Here's how the part is built. I have some questions about the finished solid (model axes, mm). A direction names the side the tool comes from. Give positions to 0.01 mm unless a question says otherwise; leave off trailing zeros. Loops run counter-clockwise (first coordinate to the right, second up) from the corner with the lowest first, then second, coordinate; pieces in that order, holes last. Notation, with made-up numbers: (57, 82.5) - (76, 82.5) arc R22 ccw to (76, 99.5) - close; hole circle Ø1 at (39, 74). An arc over 180 degrees is marked (long way). Use one line per item in the form item = value.
from build123d import *

# Parameters (mm, degrees)
SKETCH1_W           = 20
SKETCH1_H           = 60
BOSS_EXTRUDE1_DEPTH = 5
SKETCH2_W           = 20
SKETCH2_H           = 13
BOSS_EXTRUDE2_DEPTH = 4.5
SKETCH3_W           = 15
SKETCH3_H           = 6.5
CUT_EXTRUDE1_DEPTH  = 14
CUT_EXTRUDE2_DEPTH  = 10


with BuildPart() as part:
    # Sketch1 → Boss-Extrude1 (new body)
    with BuildSketch(Plane.XY):
        with Locations((10, 30)):
            Rectangle(SKETCH1_W, SKETCH1_H)
    extrude(amount=BOSS_EXTRUDE1_DEPTH)

    # Sketch2 → Boss-Extrude2 (add)
    with BuildSketch(Plane.XY.offset(5)):
        with Locations((10, 6.5)):
            Rectangle(SKETCH2_W, SKETCH2_H)
    extrude(amount=BOSS_EXTRUDE2_DEPTH)

    # Sketch3 → Cut-Extrude1 (cut, through all)
    with BuildSketch(Plane(origin=(0, 13, 0), x_dir=(1, 0, 0), z_dir=(0, 1, 0))):
        with Locations((10, -5.25)):
            Rectangle(SKETCH3_W, SKETCH3_H)
    extrude(amount=-CUT_EXTRUDE1_DEPTH, mode=Mode.SUBTRACT)

    # Sketch4 → Cut-Extrude2 (cut)
    with BuildSketch(Plane.XY.offset(5)):
        with BuildLine():
            Line((11.75, 54), (11.75, 18))
            ThreePointArc((11.75, 18), (10, 16.25), (8.25, 18))
            Line((8.25, 18), (8.25, 54))
            ThreePointArc((8.25, 54), (10, 55.75), (11.75, 54))
        make_face()
    extrude(amount=-CUT_EXTRUDE2_DEPTH, mode=Mode.SUBTRACT)


solid = part.part
(1) For faces 1 (the cylindrical face through (9.96, 55.75, 2.54)), 2 (the flat face through (10, 7, 8.5)), 3 (the flat face through (2.5, 7, 5)), which set-ups out of +Z, -Z, +X, -X, +Y, -Y let a thin tool reach every point of the face, with its end or its side?
Geometry says:
face_1 = +Z, -Z
face_2 = +Y, -Y
face_3 = -Y
(2) If I drill on probe 1 along X at (y, z) = (6.5, 3); probe 2 along X at (y, z) = (41, 0.5); probe 3 along Z at (x, y) = (8, 5), over which ranges is the centre line in solid material (lowest first)?
Geometry says:
probe_1 = 0 to 2.5, 17.5 to 20
probe_2 = 0 to 8.25, 11.75 to 20
probe_3 = 0 to 2, 8.5 to 9.5
(3) If we section it at C-C (y = 52): List the corners of the cut face in (x, z) for me, plus the area to 3 significant figures.
Geometry says:
outline = (0, 0) - (8.25, 0) - (8.25, 5) - (0, 5) - close; (11.75, 0) - (20, 0) - (20, 5) - (11.75, 5) - close
area = 82.5 mm²
(4) If we section it at A-A (x = 4.5): List the corners of the cut face in (y, z) for me.
Geometry says:
outline = (0, 0) - (60, 0) - (60, 5) - (13, 5) - (13, 2) - (0, 2) - close; (0, 8.5) - (13, 8.5) - (13, 9.5) - (0, 9.5) - close
(5) For P1, Ø6, axis at x = 12, y = 33.5, coming from the +Z side; P2, Ø1.3, axis at x = 5, z = 6.5, coming from the +Y side; P3, Ø2.5, axis at x = 6.5, z = 4, coming from the -Y side, each with a flat end and sliding along its axis, tell me the tip position at first contact or that it passes through.
Geometry says:
P1 = 5
P2 = through
P3 = 13
(6) If we section it at B-B (z = 1): List the corners of the cut face in (x, y) for me.
Geometry says:
outline = (0, 0) - (20, 0) - (20, 60) - (0, 60) - close; hole (8.25, 18) arc R1.75 ccw to (11.75, 18) - (11.75, 54) arc R1.75 ccw to (8.25, 54) - close
(7) If we section it at D-D (x = 10): List the corners of the cut face in (y, z) for me, plus the area to 3 significant figures.
Geometry says:
outline = (0, 0) - (16.25, 0) - (16.25, 5) - (13, 5) - (13, 2) - (0, 2) - close; (0, 8.5) - (13, 8.5) - (13, 9.5) - (0, 9.5) - close; (55.75, 0) - (60, 0) - (60, 5) - (55.75, 5) - close
area = 76.5 mm²
(8) Thinking about a two-plate mould opening in X: for faces 4 (the flat face through (10, 13, 3)), 5 (the flat face through (20, 23, 4)), 6 (the flat face through (0, 23, 4)), 7 (the flat face through (10, 13, 9)), which applies, pulls with the +X half, pulls with the -X half, needs draft (parallel to the pull), parting line crosses it, or undercut?
Geometry says:
face_4 = undercut
face_5 = pulls with the +X half
face_6 = pulls with the -X half
face_7 = needs draft
